```python
from build123d import *

# Parameters (mm, degrees)
F0_R     = 3.81
F0_R_2   = 6.35
F1_DEPTH = 12.7
F2_DEPTH = 6.35


with BuildPart() as f1:
    # F0 (on Top) → F1 (new body)
    with BuildSketch(Plane.XY):
        with BuildLine():
            ThreePointArc((38.735, -1.27), (34.925, 2.54), (31.115, -1.27))
            ThreePointArc((31.115, -1.27), (34.925, -5.08), (38.735, -1.27))
        make_face()
        with Locations((-34.925, -1.27)):
            Circle(F0_R)
        Polygon((-50.8, -19.05), (50.8, -19.05), (50.8, 19.05), (0, 19.05), (-50.8, 19.05), align=None)
        with Locations((-34.925, -1.27)):
            Circle(F0_R_2, mode=Mode.SUBTRACT)
        with BuildLine():
            ThreePointArc((41.275, -1.27), (34.925, -7.62), (28.575, -1.27))
            ThreePointArc((28.575, -1.27), (34.925, 5.08), (41.275, -1.27))
        make_face(mode=Mode.SUBTRACT)
        with BuildLine():
            ThreePointArc((41.275, -1.27), (34.925, 5.08), (28.575, -1.27))
            ThreePointArc((28.575, -1.27), (34.925, -7.62), (41.275, -1.27))
        make_face()
        with BuildLine():
            ThreePointArc((38.735, -1.27), (34.925, -5.08), (31.115, -1.27))
            ThreePointArc((31.115, -1.27), (34.925, 2.54), (38.735, -1.27))
        make_face(mode=Mode.SUBTRACT)
        with Locations((-34.925, -1.27)):
            Circle(F0_R_2)
        with Locations((-34.925, -1.27)):
            Circle(F0_R, mode=Mode.SUBTRACT)
    extrude(amount=-F1_DEPTH)

    # F0 (on Top) → F2 (cut)
    with BuildSketch(Plane.XY):
        with Locations((-34.925, -1.27)):
            Circle(F0_R_2)
        with Locations((-34.925, -1.27)):
            Circle(F0_R, mode=Mode.SUBTRACT)
        with BuildLine():
            ThreePointArc((41.275, -1.27), (34.925, 5.08), (28.575, -1.27))
            ThreePointArc((28.575, -1.27), (34.925, -7.62), (41.275, -1.27))
        make_face()
        with BuildLine():
            ThreePointArc((38.735, -1.27), (34.925, -5.08), (31.115, -1.27))
            ThreePointArc((31.115, -1.27), (34.925, 2.54), (38.735, -1.27))
        make_face(mode=Mode.SUBTRACT)
    extrude(amount=-F2_DEPTH, mode=Mode.SUBTRACT)


solid = f1.part
```
The listing builds one solid part. Answer for the finished solid, in the listing's coordinates (mm). A direction names the side the tool comes from. Coordinates: 2 decimals unless noted, no trailing zeros. Write each loop counter-clockwise with the first axis right and the second up, starting at its lowest first coordinate (ties: lowest second). Pieces come first, ordered by that corner, then holes. Notation, with made-up numbers: (52.25, -6.5) - (69.25, -6.5) arc R26 cw to (69.25, 22.5) - close; hole circle Ø8 at (-12, 48.25). An arc over 180 degrees is marked (long way). One line per item, written item: value.
1) Consider line 1 along X through (y, z) = (1.5, -8.25); line 2 along Y through (x, z) = (-30, -6); line 3 along Z through (x, y) = (40, 2.5). Determine where each line is inside the solid, lowest interval first. Write a range as from..to.
Geometry check:
line 1: x = -50.8..-37.54, -32.31..32.31, 37.54..50.8
line 2: y = -19.05..-5.28, 2.74..19.05
line 3: z = -12.7..-6.35
2) For a pull along X with two mould halves and no side action, classify faces 3 (the flat face through (-50.8, 0, -6)), 4 (the cylindrical face through (41.27, -1.55, -3.13)), 5 (the flat face through (-1, 0, -12.7)) as pulls with the +X half, pulls with the -X half, needs draft (parallel to the pull), parting line crosses it, or undercut.
Geometry check:
face 3: pulls with the -X half
face 4: undercut
face 5: needs draft
3) A tool of negligible diameter and unlimited length cuts with its end or side. For faces 1 (the flat face through (-32, -4, -6.35)), 2 (the flat face through (50.8, 0, -6)), from which of +Z, -Z, +X, -X, +Y, -Y can it reach the whole face along a straight path? Write none if from no direction.
Geometry check:
face 1: +Z
face 2: +Z, -Z, +X, +Y, -Y
4) Find section C-C (z = -1.5). Give the vertices of the cut face in (x, y) (3 decimals).
Geometry check:
outline: (-50.8, -19.05) - (50.8, -19.05) - (50.8, 19.05) - (-50.8, 19.05) - close; hole circle Ø12.7 at (-34.925, -1.27); hole circle Ø12.7 at (34.925, -1.27)
5) Find section A-A (y = -1.27). Give the vertices of the cut face in (x, z) (3 decimals).
Geometry check:
outline: (-50.8, -12.7) - (-38.735, -12.7) - (-38.735, -6.35) - (-41.275, -6.35) - (-41.275, 0) - (-50.8, 0) - close; (-31.115, -12.7) - (31.115, -12.7) - (31.115, -6.35) - (28.575, -6.35) - (28.575, 0) - (-28.575, 0) - (-28.575, -6.35) - (-31.115, -6.35) - close; (38.735, -12.7) - (50.8, -12.7) - (50.8, 0) - (41.275, 0) - (41.275, -6.35) - (38.735, -6.35) - close
6) Find section B-B (x = 32.5). Give the vertices of the cut face in (y, z).
Geometry check:
outline: (-19.05, -12.7) - (-4.21, -12.7) - (-4.21, -6.35) - (-7.14, -6.35) - (-7.14, 0) - (-19.05, 0) - close; (1.67, -12.7) - (19.05, -12.7) - (19.05, 0) - (4.6, 0) - (4.6, -6.35) - (1.67, -6.35) - close
7) This flat-tipped pin is pushed along its axis until it touches: pin 1 Ø9 at (x, y) = (34.925, -1.27) entering from +Z. Where does it stop, or does it pass through?
Geometry check:
pin 1: stops at z = -6.35
